Design review of the part built by this model. Coordinates are the model's own, in mm. A direction names the side the tool comes from. Give positions to 0.01 mm unless a question says otherwise; leave off trailing zeros. Loops run counter-clockwise (first coordinate to the right, second up) from the corner with the lowest first, then second, coordinate; pieces in that order, holes last. Notation, with made-up numbers: (17.5, 67) -> (30.5, 67) arc R25 cw to (30.5, 81) -> close; hole circle Ø10 at (-7.75, -1.75). An arc over 180 degrees is marked (long way). Use CSV: the item, a comma, the result in double quotes. Start each with the question number.
Item 1: We need section C-C (y = -0.75). State the section outline as (x, z) points, plus the area to 3 significant figures.
Item 2: For faces 1 (the face through (-12.805, 1, 40)), 2 (the face through (0, -10, -41)), list the 3-axis set-ups (+Z, -Z, +X, -X, +Y, -Y) from which the entire face can be reached by the end or side of a thin tool; tool diameter is ignored.
Item 3: The part is to be moulded in two halves that separate along Z. For faces 3 (the face through (34, -10, 34)), 4 (the face through (-18.283, -11.479, 44.814)), 5 (the face through (11.186, -10, -47.244)), say which applies: +Z half, -Z half, draft (parallel to the pull), parting line (faces both ways), or undercut.
Item 4: Wall thickness on line 1 along X through (y, z) = (-1, -7); line 2 along X through (y, z) = (-11.1, 0): over which ranges is each line inside the solid? List them lowest first. Write a range as from..to.
Item 5: We need section B-B (z = 11.5). State the section outline as (x, y) points, plus the area to 3 significant figures.
Item 6: We need section A-A (x = 0). State the section outline as (y, z) points, plus the area to 3 significant figures.
Item 7: Clearance check with flat-ended pins moving along their axes: pin 1 (5 mm diameter, centred on x = -40.5, z = -1.5, fed in from -Y); pin 2 (12 mm diameter, centred on x = 35, z = 1, fed in from +Y); pin 3 (4 mm diameter, centred on x = 34.5, z = -33, fed in from +Y) (3 decimals). State where each tip first meets the part, or that it passes through.
Autodesk Inventor part; units mm, degrees
ref_plane "YZ Plane" through (0, 0, 0) normal (1, 0, 0) x (0, 1, 0)
ref_plane "XZ Plane" through (0, 0, 0) normal (0, 1, 0) x (-1, 0, 0)
ref_plane "XY Plane" through (0, 0, 0) normal (0, 0, 1) x (1, 0, 0)
sketch "Sketch1" plane through (0, 0, 0) normal (0, 1, 0) x (-1, 0, 0)
  line L0 (49.3, -49.3) -> (-49.3, -49.3)
  line L1 (-49.3, -49.3) -> (-49.3, 49.3)
  line L2 (-49.3, 49.3) -> (49.3, 49.3)
  line L3 (49.3, 49.3) -> (49.3, -49.3)
  line L4 (49.3, -49.3) -> (-49.3, 49.3) construction
  line L5 (-49.3, -49.3) -> (49.3, 49.3) construction
  line L6 (48.4, -48.4) -> (-48.4, -48.4)
  line L7 (-48.4, -48.4) -> (-48.4, 48.4)
  line L8 (-48.4, 48.4) -> (48.4, 48.4)
  line L9 (48.4, 48.4) -> (48.4, -48.4)
  line L10 (48.4, -48.4) -> (-48.4, 48.4) construction
  line L11 (-48.4, -48.4) -> (48.4, 48.4) construction
  line L12 (38.4, -38.4) -> (-38.4, -38.4)
  line L13 (-38.4, -38.4) -> (-38.4, 38.4)
  line L14 (-38.4, 38.4) -> (38.4, 38.4)
  line L15 (38.4, 38.4) -> (38.4, -38.4)
  line L16 (38.4, -38.4) -> (-38.4, 38.4) construction
  line L17 (-38.4, -38.4) -> (38.4, 38.4) construction
  line L18 (37.4, -37.4) -> (-37.4, -37.4)
  line L19 (-37.4, -37.4) -> (-37.4, 37.4)
  line L20 (-37.4, 37.4) -> (37.4, 37.4)
  line L21 (37.4, 37.4) -> (37.4, -37.4)
  line L22 (37.4, -37.4) -> (-37.4, 37.4) construction
  line L23 (-37.4, -37.4) -> (37.4, 37.4) construction
  line L24 (24.3286, 38.4) -> (24.3286, 48.4)
  line L25 (24.3286, 38.4) -> (23.3286, 38.4)
  line L26 (23.3286, 38.4) -> (23.3286, 48.4)
  line L27 (24.3286, 48.4) -> (23.3286, 48.4)
  circle A0 centre (17.6595, 43.4) radius 3.4806
  line L28 (12.8049, 38.4) -> (12.8049, 41.4)
  line L29 (12.8049, 41.4) -> (11.8049, 41.4)
  line L30 (11.8049, 41.4) -> (11.8049, 38.4)
  line L31 (12.8049, 48.4) -> (12.8049, 45.4)
  line L32 (12.8049, 45.4) -> (11.8049, 45.4)
  line L33 (11.8049, 45.4) -> (11.8049, 48.4)
  point P0 (0, 0)
  dimension "d0" = 98.6
  dimension "d1" = 98.6
  dimension "d2" = 96.8
  dimension "d3" = 96.8
  dimension "d4" = 76.8
  dimension "d5" = 76.8
  dimension "d6" = 74.8
  dimension "d7" = 74.8
  dimension "d8" = 10
  dimension "d9" = 1
  dimension "d10" = 3
  dimension "d11" = 1
  dimension "d12" = 3
extrude "Extrusion1" add sketch "Sketch1" along normal mid plane 20 contours L0 L1 L2 L3 | L6 L7 L8 L33 L32 L31 L26 L14 L28 L29 L30 L13 L12 L15 L24 L9 | L24 L14 L26 L8 | L8 L31 L32 L33 | L14 L15 L12 L13 | L14 L30 L29 L28 | L18 L19 L20 L21 | A0
extrude "Extrusion2" cut sketch "Sketch1" along normal mid plane 29.525 contours L18 L19 L20 L21
extrude "Extrusion3" cut sketch "Sketch1" along normal blind 29.525 and the other way blind 8 contours L6 L7 L8 L33 L32 L31 L26 L14 L28 L29 L30 L13 L12 L15 L24 L9
extrude "Extrusion4" cut sketch "Sketch1" along normal blind 29.525 and the other way blind 14.763 contours A0
sketch "Sketch2" plane through (0, -10, 0) normal (0, -1, 0) x (1, 0, 0)
  arc A0 (40.1076, -27.0913) -> (-15.2678, 45.9288) centre (0, 0) ccw
  arc A1 (-14.6167, 45.09) -> (-14.6288, 45.0861) centre (0, 0) ccw
  circle A2 centre (-17.6595, 43.4) radius 3.4806
  line L0 (-14.6288, 45.0861) -> (-14.5793, 45.0208)
  circle A3 centre (0, 0) radius 47.4
  arc A4 (-15.2678, 45.9288) -> (-21.1372, 43.5405) centre (0, 0) ccw
  circle A5 centre (0, 0) radius 48.4
  arc A6 (-14.5793, 45.0208) -> (-14.6167, 45.09) centre (-17.6595, 43.4) ccw
  arc A7 (-15.2678, 45.9288) -> (-21.1372, 43.5405) centre (-17.6595, 43.4) ccw
  point P0 (-14.6167, 45.09)
  point P1 (-15.2678, 45.9288)
  point P2 (-14.6167, 45.09)
  dimension "d25" = 96.8
  dimension "d26" = 94.8
sketch "Sketch3" plane through (0, -10, 0) normal (0, -1, 0) x (1, 0, 0)
  arc A0 (-21.1372, 43.5405) -> (-15.2678, 45.9288) centre (0, 0) ccw
  line L0 (37.4, -37.4) -> (37.4, 37.4)
  line L1 (37.4, -29.1204) -> (37.4, -30.7213)
  line L2 (37.4, -30.7213) -> (37.4, -37.4)
  line L3 (37.4, -37.4) -> (-37.4, -37.4)
  line L4 (37.4, -37.4) -> (30.7213, -37.4)
  arc A1 (-37.4, -30.7213) -> (-30.7213, -37.4) centre (0, 0) ccw
  line L5 (-37.4, -37.4) -> (-30.7213, -37.4)
  arc A2 (-37.4, 30.7213) -> (-37.4, -30.7213) centre (0, 0) ccw
  line L6 (-37.4, -37.4) -> (-37.4, -30.7213)
  line L7 (-37.4, 37.4) -> (-37.4, -37.4)
  line L8 (-37.4, 30.7213) -> (-37.4, 37.4)
  line L9 (-37.4, 37.4) -> (37.4, 37.4)
  line L10 (-37.4, 37.4) -> (-30.7213, 37.4)
  arc A3 (37.4, 30.7213) -> (30.7213, 37.4) centre (0, 0) ccw
  line L11 (37.4, 37.4) -> (37.4, -37.4)
  line L12 (37.4, 30.7213) -> (37.4, 37.4)
  line L13 (-37.4, 37.4) -> (37.4, 37.4)
  line L14 (37.4, 37.4) -> (30.7213, 37.4)
  arc A4 (30.7213, -37.4) -> (37.4, -30.7213) centre (0, 0) ccw
  arc A5 (-37.4, -30.7213) -> (-30.7213, -37.4) centre (0, 0) ccw
  arc A6 (37.4, 30.7213) -> (30.7213, 37.4) centre (0, 0) ccw
  arc A7 (-30.7213, 37.4) -> (-37.4, 30.7213) centre (0, 0) ccw
  point P0 (37.4, 30.7213)
  point P1 (37.4, -30.7213)
extrude "Extrusion6" add sketch "Sketch3" against normal blind 0.175 contours A0 L7 L9 | L9 L0 A0 | A0 L3 L6 | L0 L3 A0
extrude "Extrusion8" add sketch "Sketch2" against normal blind 0.175 contours A2 A4
extrude "Extrusion9" add sketch "Sketch2" along normal blind 3 contours A5 A2 A3 A0 | A4 A2 A1 A3
Results found:
1,outline,"(-49.3, -49.3) -> (49.3, -49.3) -> (49.3, 49.3) -> (-49.3, 49.3) -> close; hole (-48.4, -48.4) -> (48.4, -48.4) -> (48.4, 48.4) -> (-11.8, 48.4) -> (-11.8, 45.4) -> (-12.8, 45.4) -> (-12.8, 48.4) -> (-23.33, 48.4) -> (-23.33, 38.4) -> (-12.8, 38.4) -> (-12.8, 41.4) -> (-11.8, 41.4) -> (-11.8, 38.4) -> (38.4, 38.4) -> (38.4, -38.4) -> (-38.4, -38.4) -> (-38.4, 38.4) -> (-24.33, 38.4) -> (-24.33, 48.4) -> (-48.4, 48.4) -> close; hole (-37.4, -37.4) -> (37.4, -37.4) -> (37.4, 37.4) -> (-37.4, 37.4) -> close"
1,area,"671 mm²"
2,face 1,"+Y"
2,face 2,"-Y"
3,face 3,"undercut"
3,face 4,"+Z half"
3,face 5,"draft"
4,line 1,"-49.3..-48.4, -38.4..-37.4, 37.4..38.4, 48.4..49.3"
4,line 2,"-48.4..-47.4, 47.4..48.4"
5,outline,"(-49.3, -10) -> (-47.01, -10) -> (-47.01, -13) -> (-45.98, -13) -> (-45.98, -10) -> (-37.4, -10) -> (-37.4, 10) -> (-38.4, 10) -> (-38.4, -8) -> (-48.4, -8) -> (-48.4, 10) -> (-49.3, 10) -> close; (37.4, -10) -> (45.98, -10) -> (45.98, -13) -> (47.01, -13) -> (47.01, -10) -> (49.3, -10) -> (49.3, 10) -> (48.4, 10) -> (48.4, -8) -> (38.4, -8) -> (38.4, 10) -> (37.4, 10) -> close"
5,area,"122 mm²"
6,outline,"(-13, -48.4) -> (-10, -48.4) -> (-10, -49.3) -> (10, -49.3) -> (10, -48.4) -> (-8, -48.4) -> (-8, -38.4) -> (10, -38.4) -> (10, -37.4) -> (-10, -37.4) -> (-10, -47.4) -> (-13, -47.4) -> close; (-13, 47.4) -> (-10, 47.4) -> (-10, 37.4) -> (10, 37.4) -> (10, 38.4) -> (-8, 38.4) -> (-8, 48.4) -> (10, 48.4) -> (10, 49.3) -> (-10, 49.3) -> (-10, 48.4) -> (-13, 48.4) -> close"
6,area,"122 mm²"
7,pin 1,"y = -10"
7,pin 2,"y = 10"
7,pin 3,"y = -9.825"
